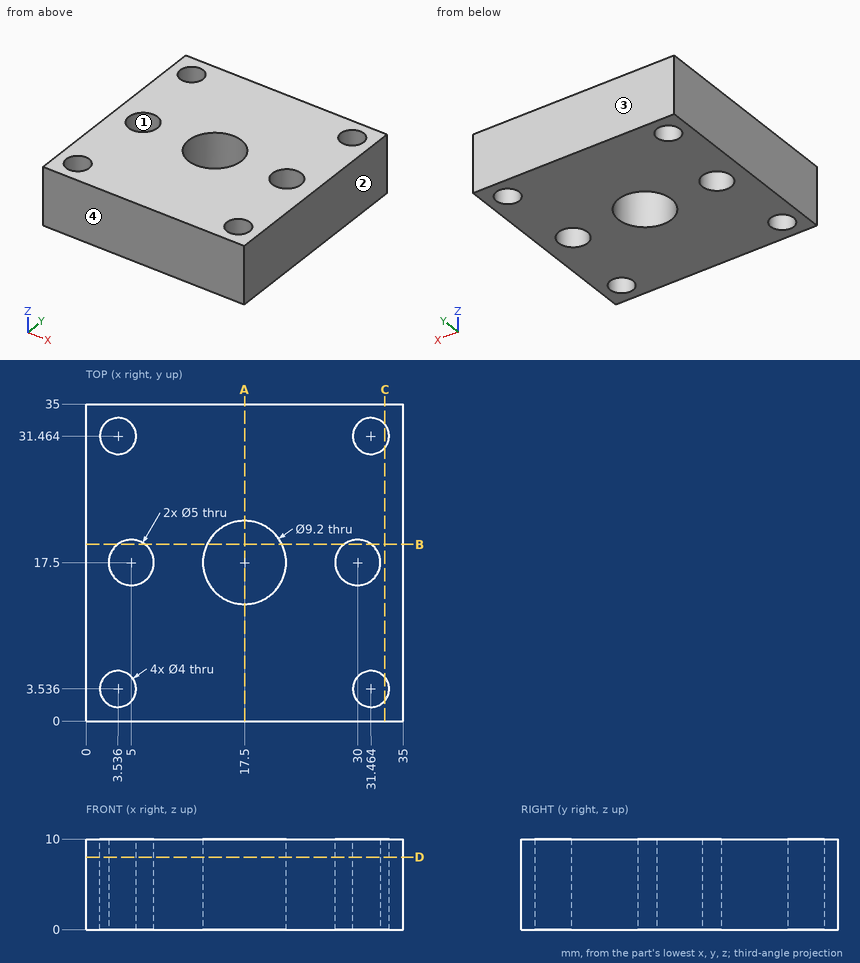
Could you check a few things on this drawing? It's one solid part, dimensions in mm from its lowest x, y, z. Round coordinates to 2 decimals unless told otherwise and drop trailing zeros. Order: outer loops, then holes, each group sorted by start corner. A loop starts at its lowest first (then second) coordinate and runs counter-clockwise, first axis right, second up. Notation, with made-up numbers: M 83.25,-27.5 L 135.25,-27.5 A26 cw 135.25,1.5 Z; hole C 30.5,85.25 d9. An arc over 180 degrees is marked long. One line per item, written item: value.
(1) Imagine slicing it at A-A (x = 17.5). Write out the boundary of the cut face in (y, z), and give its area (3 significant figures).
Ans:
outline: M 0,0 L 12.9,0 L 12.9,10 L 0,10 Z; M 22.1,0 L 35,0 L 35,10 L 22.1,10 Z
area: 258 mm^2
(2) Imagine slicing it at D-D (z = 8). Write out the boundary of the cut face in (x, y) (1 decimal).
Ans:
outline: M 0,0 L 35,0 L 35,35 L 0,35 Z; hole C 3.5,3.5 d4; hole C 3.5,31.5 d4; hole C 5,17.5 d5; hole C 17.5,17.5 d9.2; hole C 30,17.5 d5; hole C 31.5,3.5 d4; hole C 31.5,31.5 d4
(3) Imagine slicing it at B-B (y = 19.5). Write out the boundary of the cut face in (x, z).
Ans:
outline: M 0,0 L 3.5,0 L 3.5,10 L 0,10 Z; M 6.5,0 L 13.36,0 L 13.36,10 L 6.5,10 Z; M 21.64,0 L 28.5,0 L 28.5,10 L 21.64,10 Z; M 31.5,0 L 35,0 L 35,10 L 31.5,10 Z
(4) I need wall thicknesses on line 1 along Y through (x, z) = (17.5, 7.75); line 2 along Y through (x, z) = (30, 3.75) (1 decimal); line 3 along Y through (x, z) = (31.5, 2) (1 decimal). Which ranges of each line are inside material? Lowest first, please. Write a range as from..to.
Ans:
line 1: y = 0..12.9, 22.1..35
line 2: y = 0..2.2, 4.9..15, 20..30.1, 32.8..35
line 3: y = 0..1.5, 5.5..15.5, 19.5..29.5, 33.5..35
(5) If we mould it in two halves opening along Y, with no side actions, what happens to the marked faces 1, 2, 3 and 4? For each: released by +Y, released by -Y, zero draft, split by the parting line, or undercut.
Ans:
face 1: undercut
face 2: zero draft
face 3: released by +Y
face 4: released by -Y
(6) Imagine slicing it at C-C (x = 33). Write out the boundary of the cut face in (y, z) (1 decimal).
Ans:
outline: M 0,0 L 2.3,0 L 2.3,10 L 0,10 Z; M 4.8,0 L 30.2,0 L 30.2,10 L 4.8,10 Z; M 32.7,0 L 35,0 L 35,10 L 32.7,10 Z
(7) I'm going to push flat-ended pins straight in: P1, Ø3, axis at x = 31.46, y = 31.46, coming from the -Z side; P2, Ø4.5, axis at x = 3.54, y = 31.46, coming from the -Z side. Where does each tip first touch, or does it pass through?
Ans:
P1: passes through
P2: stops at z = 0
